Autodesk Inventor part; units mm, degrees
ref_plane "YZ Plane" through (0, 0, 0) normal (1, 0, 0) x (0, 1, 0)
ref_plane "XZ Plane" through (0, 0, 0) normal (0, 1, 0) x (-1, 0, 0)
ref_plane "XY Plane" through (0, 0, 0) normal (0, 0, 1) x (1, 0, 0)
sketch "Sketch1" plane through (0, 0, 0) normal (0, 0, 1) x (1, 0, 0)
  line L0 (0, -13.8137) -> (15, -13.8137)
  line L1 (0, 0) -> (0, -13.8137)
  line L2 (45, 0) -> (0, 0)
  line L3 (45, 0) -> (45, -13.8137)
  line L4 (30, -13.8137) -> (45, -13.8137)
  line L5 (30, -6) -> (30, -13.8137)
  line L6 (30, -6) -> (15, -6)
  line L7 (15, -6) -> (15, -13.8137)
  line L8 (-2.5, 0) -> (-2.5, -11.3137)
  line L9 (47.5, 0) -> (-2.5, 0)
  line L10 (47.5, 0) -> (75, 32.7732)
  line L11 (47.5, 0) -> (90.2824, 0) construction
  line L12 (75, 32.7732) -> (75, 72.7732)
  line L13 (75, 72.7732) -> (52.5, 80.9626)
  line L14 (52.5, 80.9626) -> (52.5, 110.5752)
  line L15 (22.5, -6) -> (22.5, 110.5752)
  line L16 (-10.9317, 221.1504) -> (1.7683, 221.1504) construction
  line L17 (22.5, 0) -> (22.5, 221.1504)
  line L18 (22.5, 110.5752) -> (52.5, 110.5752) construction
  line L19 (-2.5, 0) -> (-30, 32.7732)
  line L20 (-30, 32.7732) -> (-30, 72.7732)
  line L21 (-30, 72.7732) -> (-7.5, 80.9626)
  line L22 (-7.5, 80.9626) -> (2.5, 84.6023)
  line L23 (2.5, 84.6023) -> (2.5, 110.5752)
  line L24 (22.5, 110.5752) -> (2.5, 110.5752) construction
  line L25 (47.5, 221.1504) -> (75, 188.3772)
  line L26 (75, 188.3772) -> (75, 148.3772)
  line L27 (75, 148.3772) -> (52.5, 140.1879)
  line L28 (52.5, 140.1879) -> (52.5, 110.5752)
  line L29 (-30, 148.3772) -> (-7.5, 140.1879)
  line L30 (-30, 188.3772) -> (-30, 148.3772)
  line L31 (-2.5, 221.1504) -> (-30, 188.3772)
  line L32 (-7.5, 140.1879) -> (2.5, 136.5482)
  line L33 (2.5, 136.5482) -> (2.5, 110.5752)
  line L34 (0, 234.9641) -> (15, 234.9641)
  line L35 (0, 221.1504) -> (0, 234.9641)
  line L36 (45, 221.1504) -> (45, 234.9641)
  line L37 (30, 234.9641) -> (45, 234.9641)
  line L38 (30, 227.1504) -> (30, 234.9641)
  line L39 (30, 227.1504) -> (15, 227.1504)
  line L40 (15, 227.1504) -> (15, 234.9641)
  line L41 (47.5, 221.1504) -> (-2.5, 221.1504)
  line L42 (75, 40) -> (75, 44.6908)
  dimension "d0" = 50
  dimension "d1" = 110
  dimension "d2" = 30
  dimension "d3" = 40
  dimension "d4" = 30
  dimension "d5" = 20
extrude "Extrusion1" add sketch "Sketch1" along normal blind 3
sketch "Sketch2" plane through (0, 0, 3) normal (0, 0, 1) x (1, 0, 0)
  line L0 (45, -13.8137) -> (45, 0)
  line L1 (45, 0) -> (47.5, 0)
  line L2 (47.5, 0) -> (75, 32.7732)
  line L3 (75, 32.7732) -> (75, 72.7732)
  line L4 (75, 72.7732) -> (52.5, 80.9626)
  line L5 (52.5, 80.9626) -> (52.5, 140.1879)
  line L6 (52.5, 140.1879) -> (75, 148.3772)
  line L7 (75, 148.3772) -> (75, 188.3772)
  line L8 (75, 188.3772) -> (47.5, 221.1504)
  line L9 (47.5, 221.1504) -> (45, 221.1504)
  line L10 (45, 221.1504) -> (45, 234.9641)
  line L11 (45, 234.9641) -> (30, 234.9641)
  line L12 (30, 234.9641) -> (30, 227.1504)
  line L13 (30, 227.1504) -> (15, 227.1504)
  line L14 (15, 227.1504) -> (15, 234.9641)
  line L15 (15, 234.9641) -> (0, 234.9641)
  line L16 (0, 234.9641) -> (0, 221.1504)
  line L17 (0, 221.1504) -> (-2.5, 221.1504)
  line L18 (-2.5, 221.1504) -> (-30, 188.3772)
  line L19 (-30, 188.3772) -> (-30, 148.3772)
  line L20 (-30, 148.3772) -> (2.5, 136.5482)
  line L21 (2.5, 136.5482) -> (2.5, 84.6023)
  line L22 (2.5, 84.6023) -> (-30, 72.7732)
  line L23 (-30, 72.7732) -> (-30, 32.7732)
  line L24 (-30, 32.7732) -> (-2.5, 0)
  line L25 (-2.5, 0) -> (0, 0)
  line L26 (0, 0) -> (0, -13.8137)
  line L27 (0, -13.8137) -> (15, -13.8137)
  line L28 (15, -13.8137) -> (15, -6)
  line L29 (15, -6) -> (30, -6)
  line L30 (30, -6) -> (30, -13.8137)
  line L31 (30, -13.8137) -> (45, -13.8137)
  line L32 (-20, 36.4129) -> (-20, 65.7711)
  line L33 (-20, 65.7711) -> (12.5, 77.6002)
  line L34 (12.5, 77.6002) -> (12.5, 143.5503)
  line L35 (12.5, 143.5503) -> (-20, 155.3793)
  line L36 (-20, 155.3793) -> (-20, 184.7375)
  line L37 (-20, 184.7375) -> (2.1631, 211.1504)
  line L38 (2.1631, 211.1504) -> (10, 211.1504)
  line L39 (10, 211.1504) -> (10, 217.1504)
  line L40 (10, 217.1504) -> (35, 217.1504)
  line L41 (35, 217.1504) -> (35, 211.1504)
  line L42 (35, 211.1504) -> (42.8369, 211.1504)
  line L43 (42.8369, 211.1504) -> (65, 184.7375)
  line L44 (65, 184.7375) -> (65, 155.3793)
  line L45 (65, 155.3793) -> (42.5, 147.19)
  line L46 (42.5, 147.19) -> (42.5, 73.9605)
  line L47 (42.5, 73.9605) -> (65, 65.7711)
  line L48 (65, 65.7711) -> (65, 36.4129)
  line L49 (65, 36.4129) -> (42.8369, 10)
  line L50 (42.8369, 10) -> (35, 10)
  line L51 (35, 10) -> (35, 4)
  line L52 (35, 4) -> (10, 4)
  line L53 (10, 4) -> (10, 10)
  line L54 (10, 10) -> (2.1631, 10)
  line L55 (2.1631, 10) -> (-20, 36.4129)
  line L56 (12.5, 77.6002) -> (12.5, 10)
  line L57 (12.5, 10) -> (10, 10)
  line L58 (22.5, 4) -> (22.5, 217.1504) construction
  line L59 (32.5, 77.6002) -> (32.5, 10)
  line L60 (32.5, 10) -> (35, 10)
  line L61 (32.5, 77.6002) -> (32.5, 211.1504)
  line L62 (32.5, 211.1504) -> (35, 211.1504)
  line L63 (12.5, 143.5503) -> (12.5, 211.1504)
  line L64 (12.5, 211.1504) -> (10, 211.1504)
  line L65 (-20, 55.1294) -> (12.5, 66.9584)
  line L66 (-25.1903, 42.5985) -> (12.5, 56.3166)
  line L67 (-18.3499, 34.4464) -> (12.5, 45.6748)
  line L68 (-11.5095, 26.2943) -> (12.5, 35.0331)
  line L69 (-4.6691, 18.1423) -> (12.5, 24.3913)
  line L70 (65, 55.1294) -> (32.5, 66.9584)
  line L71 (70.1903, 42.5985) -> (32.5, 56.3166)
  line L72 (63.3499, 34.4464) -> (32.5, 45.6748)
  line L73 (56.5095, 26.2943) -> (32.5, 35.0331)
  line L74 (49.6691, 18.1423) -> (32.5, 24.3913)
  line L75 (42.5, 73.9605) -> (32.5, 77.6002)
  point P0 (32.5, 66.9584)
  point P1 (65, 55.1294)
  point P2 (73.2901, 46.2927)
  point P3 (32.5, 56.3166)
  point P4 (32.5, 45.6748)
  point P5 (63.3499, 34.4464)
  point P6 (56.5095, 26.2943)
  point P7 (32.5, 35.0331)
  point P8 (32.5, 24.3913)
  point P9 (49.6691, 18.1423)
  point P10 (65, 44.4876)
  point P11 (-20, 44.4876)
  dimension "d8" = 10
  dimension "d9" = 10
  dimension "d10" = 10
  dimension "d11" = 10
  dimension "d12" = 10
  dimension "d13" = 10
extrude "Extrusion2" cut sketch "Sketch2" against normal blind 3 contours L32 L33 L56 L65 | L66 L56 L67 L55 L32 | L68 L56 L69 L55 | L75 L47 L48 L70 L59 | L71 L48 L49 L72 L59 | L74 L59 L73 L49
ref_plane "Work Plane1" through (0, 110.5752, 0) normal (0, 1, 0) x (1, 0, 0)
mirror "Mirror1" about plane through (0, 110.5752, 0) normal (0, 1, 0) of "Extrusion2"
sketch "Sketch3" plane through (0, 0, 0) normal (0, 0, -1) x (-1, 0, 0)
  line L0 (4.6691, 203.0082) -> (11.5095, 194.8561)
  line L1 (-32.5, 143.5503) -> (-65, 155.3793)
  line L2 (-65, 155.3793) -> (-65, 166.0211)
  line L3 (-56.5095, 194.8561) -> (-49.6691, 203.0082)
  line L4 (20, 166.0211) -> (20, 155.3793)
  line L5 (20, 155.3793) -> (-12.5, 143.5503)
  line L6 (11.5095, 26.2943) -> (4.6691, 18.1423)
  line L7 (-65, 55.1294) -> (-65, 65.7711)
  line L8 (-65, 65.7711) -> (-32.5, 77.6002)
  line L9 (-49.6691, 18.1423) -> (-56.5095, 26.2943)
  line L10 (-12.5, 77.6002) -> (20, 65.7711)
  line L11 (20, 65.7711) -> (20, 55.1294)
  line L12 (-45, -13.8137) -> (-45, 0)
  line L13 (-30, -13.8137) -> (-45, -13.8137)
  line L14 (-30, -6) -> (-30, -13.8137)
  line L15 (-15, -6) -> (-30, -6)
  line L16 (-15, -13.8137) -> (-15, -6)
  line L17 (0, -13.8137) -> (-15, -13.8137)
  line L18 (0, 0) -> (0, -13.8137)
  line L19 (2.5, 0) -> (0, 0)
  line L20 (30, 32.7732) -> (2.5, 0)
  line L21 (30, 72.7732) -> (30, 32.7732)
  line L22 (-2.5, 84.6023) -> (30, 72.7732)
  line L23 (-2.5, 136.5482) -> (-2.5, 84.6023)
  line L24 (30, 148.3772) -> (-2.5, 136.5482)
  line L25 (30, 188.3772) -> (30, 148.3772)
  line L26 (2.5, 221.1504) -> (30, 188.3772)
  line L27 (0, 221.1504) -> (2.5, 221.1504)
  line L28 (0, 234.9641) -> (0, 221.1504)
  line L29 (-15, 234.9641) -> (0, 234.9641)
  line L30 (-15, 227.1504) -> (-15, 234.9641)
  line L31 (-30, 227.1504) -> (-15, 227.1504)
  line L32 (-30, 234.9641) -> (-30, 227.1504)
  line L33 (-45, 234.9641) -> (-30, 234.9641)
  line L34 (-45, 221.1504) -> (-45, 234.9641)
  line L35 (-47.5, 221.1504) -> (-45, 221.1504)
  line L36 (-75, 188.3772) -> (-47.5, 221.1504)
  line L37 (-75, 148.3772) -> (-75, 188.3772)
  line L38 (-52.5, 140.1879) -> (-75, 148.3772)
  line L39 (-52.5, 80.9626) -> (-52.5, 140.1879)
  line L40 (-75, 72.7732) -> (-52.5, 80.9626)
  line L41 (-75, 32.7732) -> (-75, 72.7732)
  line L42 (-47.5, 0) -> (-75, 32.7732)
  line L43 (-45, 0) -> (-47.5, 0)
  circle A0 centre (25, 67.7732) radius 1.75
  circle A1 centre (25, 57.7732) radius 1.75
  circle A2 centre (25, 47.7732) radius 1.75
  line L44 (-2.5, 136.5482) -> (-2.5, 84.6023)
  line L45 (-2.5, 110.5752) -> (-52.5, 110.5752)
  circle A3 centre (25, 153.3772) radius 1.75
  circle A4 centre (25, 163.3772) radius 1.75
  circle A5 centre (25, 173.3772) radius 1.75
  line L46 (-15, -6) -> (-30, -6)
  line L47 (-22.5, -6) -> (-22.5, 227.1504)
  line L48 (-30, 227.1504) -> (-15, 227.1504)
  circle A6 centre (-70, 67.7732) radius 1.75
  circle A7 centre (-70, 57.7732) radius 1.75
  circle A8 centre (-70, 47.7732) radius 1.75
  circle A9 centre (-70, 153.3772) radius 1.75
  circle A10 centre (-70, 163.3772) radius 1.75
  circle A11 centre (-70, 173.3772) radius 1.75
  line L49 (-12.5, 154.192) -> (20, 166.0211)
  line L50 (-12.5, 143.5503) -> (-12.5, 154.192)
  line L51 (-49.6691, 203.0082) -> (-32.5, 196.7591)
  line L52 (-32.5, 196.7591) -> (-32.5, 186.1174)
  line L53 (-32.5, 186.1174) -> (-56.5095, 194.8561)
  line L54 (-32.5, 154.192) -> (-32.5, 143.5503)
  line L55 (-65, 166.0211) -> (-32.5, 154.192)
  line L56 (11.5095, 194.8561) -> (-12.5, 186.1174)
  line L57 (-12.5, 186.1174) -> (-12.5, 196.7591)
  line L58 (-12.5, 196.7591) -> (4.6691, 203.0082)
  line L59 (20, 55.1294) -> (-12.5, 66.9584)
  line L60 (-12.5, 66.9584) -> (-12.5, 77.6002)
  line L61 (-32.5, 24.3913) -> (-49.6691, 18.1423)
  line L62 (-56.5095, 26.2943) -> (-32.5, 35.0331)
  line L63 (-32.5, 35.0331) -> (-32.5, 24.3913)
  line L64 (-32.5, 77.6002) -> (-32.5, 66.9584)
  line L65 (-32.5, 66.9584) -> (-65, 55.1294)
  line L66 (-12.5, 35.0331) -> (11.5095, 26.2943)
  line L67 (4.6691, 18.1423) -> (-12.5, 24.3913)
  line L68 (-12.5, 24.3913) -> (-12.5, 35.0331)
  dimension "d16" = 3.5
  dimension "d19" = 10
  dimension "d24" = 5
  dimension "d25" = 5
extrude "Extrusion3" cut sketch "Sketch3" against normal through all contours A0 | A1 | A2 | A3 | A4 | A5 | A6 | A7 | A8 | A9 | A10 | A11
properties part number "Backplane"
Geometry check sheet. Reference: the model listing, model coordinates, mm. A direction names the side the tool comes from. Coordinates: 2 decimals unless noted, no trailing zeros. Order: outer loops, then holes, each group sorted by start corner. A loop starts at its lowest first (then second) coordinate and runs counter-clockwise, first axis right, second up. Notation, with made-up numbers: (2.25, 76.5) - (58.25, 76.5) arc R19 ccw to (58.25, 97.5) - close; hole circle Ø3 at (8, 19.5). An arc over 180 degrees is marked (long way). Answer as a JSON object with one key per item and string values. Group by question number.
Item 1: Scan lines: probe 1 along Y at (x, z) = (29, 1.2); probe 2 along X at (y, z) = (96.5, 2.4). Record each from-to range of solid material in increasing order.
Item 2: Sectioned sample at B-B, the plane z = 1.2. Give the number of separate pieces and of enclosed holes in the cut face, and give its area (3 significant figures).
Item 3: Depth check by flat-ended pin: pin 1 Ø3 at (x, y) = (-25, 173.38) entering from +Z; pin 2 Ø1.2 at (x, z) = (-1, 2) entering from +Y. Enter the tip coordinate at first touch or a pass-through.
Item 4: Sectioned sample at A-A, the plane y = 119. Record the cut outline in (x, z).
Item 5: Draft check along Y on faces 1 (the face through (48.98, 50.32, 1.52)), 2 (the face through (-16.06, 16.16, 1.48)), 3 (the face through (22, 112, 0)). Enter one of: +Y half, -Y half, draft (parallel to the pull), parting line (faces both ways), or undercut.
Item 6: Tool access check on faces 4 (the face through (-3.523, 160.024, 1.521)), 5 (the face through (61.06, 204.99, 1.48)), 6 (the face through (63.91, 76.81, 1.48)). Record the directions out of +Z, -Z, +X, -X, +Y, -Y that give a thin tool (end or side, any length) a straight path to the whole face; none if there is none.
Resolved:
{
 "1": {"probe 1": "-6 to 227.15", "probe 2": "2.5 to 52.5"},
 "2": {"separate pieces": "1", "enclosed holes": "24", "area": "15,100 mm^2"},
 "3": {"pin 1": "through", "pin 2": "y = 221.15"},
 "4": {"outline": "(2.5, 0) - (52.5, 0) - (52.5, 3) - (2.5, 3) - close"},
 "5": {"face 1": "undercut", "face 2": "-Y half", "face 3": "draft"},
 "6": {"face 4": "+Z, -Z", "face 5": "+Z, -Z, +X, +Y", "face 6": "+Z, -Z, +X"}
}
